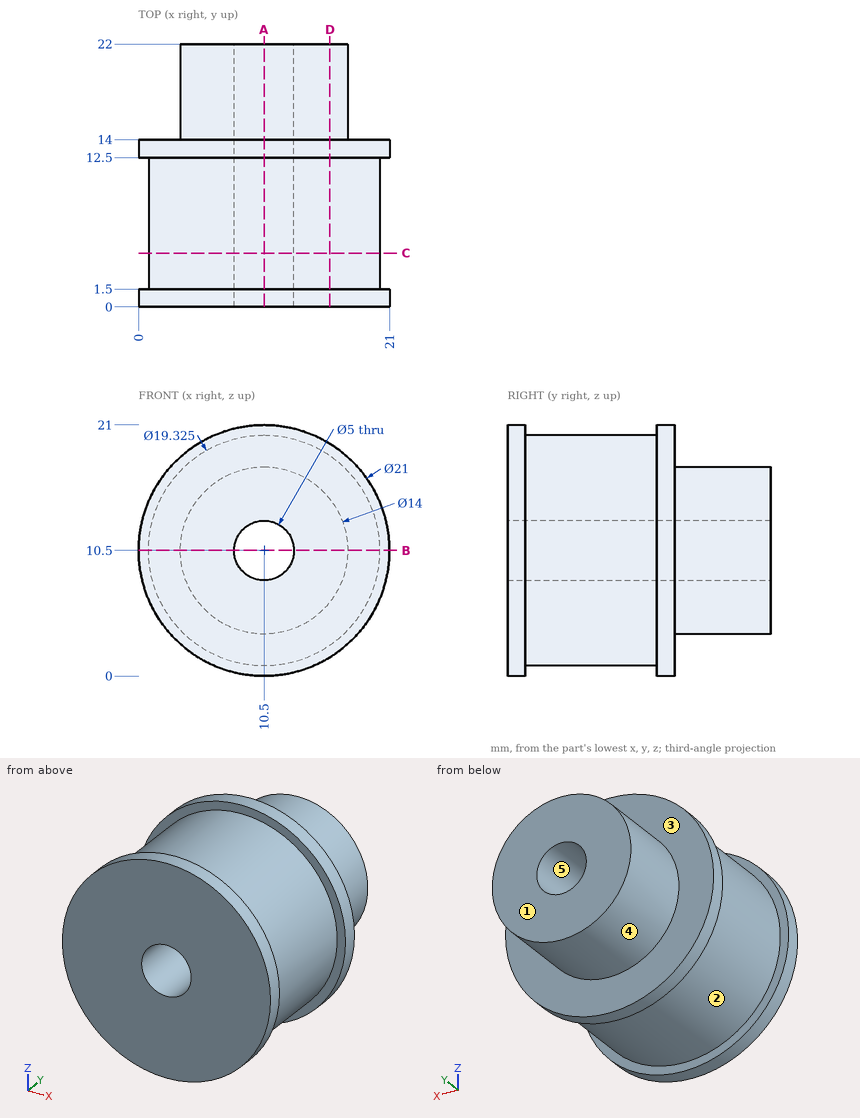
The drawing under review shows one solid part. Ordinate dimensions are in mm from its lowest x, y, z. A direction names the side the tool comes from. Coordinates: 2 decimals unless noted, no trailing zeros. Order: outer loops, then holes, each group sorted by start corner. A loop starts at its lowest first (then second) coordinate and runs counter-clockwise, first axis right, second up. Notation, with made-up numbers: (52, 31.5) -> (56, 31.5) arc R23 cw to (56, 67.5) -> close; hole circle Ø7 at (74.5, 54.25). An arc over 180 degrees is marked (long way). Use CSV: the item, a comma, the result in double quotes. Start each with the question number.
Item 1: We need section A-A, the plane x = 10.5. Give the boundary of the cut face in (y, z).
Item 2: We need section D-D, the plane x = 16. Give the boundary of the cut face in (y, z).
Item 3: We need section C-C, the plane y = 4.5. Give the boundary of the cut face in (x, z) (1 decimal), then the cut area to 3 significant figures.
Item 4: We need section B-B, the plane z = 10.5. Give the boundary of the cut face in (x, y).
Item 5: For the marked faces 1 and 2, list the 3-axis set-ups (+Z, -Z, +X, -X, +Y, -Y) from which the entire face can be reached by the end or side of a thin tool; tool diameter is ignored.
Item 6: Wall thickness on probe 1 along X at (y, z) = (5.25, 10.5); probe 2 along X at (y, z) = (13.25, 10.5); probe 3 along X at (y, z) = (16.5, 14.75): over which ranges is each line inside the solid? List them lowest first.
Item 7: Insertion check: pin 1 (3 mm diameter, centred on y = 10.5, z = 3, fed in from +X); pin 2 (1 mm diameter, centred on x = 11, z = 10, fed in from +Y); pin 3 (8 mm diameter, centred on x = 2.5, y = 17, fed in from -Z); pin 4 (1.5 mm diameter, centred on x = 10.5, y = 8, fed in from -Z). Each pin has a flat end and moves straight along its axis. Give the tip position at first contact, or say it passes through.
Item 8: Draft analysis for pull direction X (two halves, no side actions). For the marked faces 3, 4 and 5, state which applies: pulls with the +X half, pulls with the -X half, needs draft (parallel to the pull), parting line crosses it, or undercut.
Derived:
1,outline,"(0, 0) -> (1.5, 0) -> (1.5, 0.84) -> (12.5, 0.84) -> (12.5, 0) -> (14, 0) -> (14, 3.5) -> (22, 3.5) -> (22, 8) -> (0, 8) -> close; (0, 13) -> (22, 13) -> (22, 17.5) -> (14, 17.5) -> (14, 21) -> (12.5, 21) -> (12.5, 20.16) -> (1.5, 20.16) -> (1.5, 21) -> (0, 21) -> close"
2,outline,"(0, 1.56) -> (1.5, 1.56) -> (1.5, 2.56) -> (12.5, 2.56) -> (12.5, 1.56) -> (14, 1.56) -> (14, 6.17) -> (22, 6.17) -> (22, 14.83) -> (14, 14.83) -> (14, 19.44) -> (12.5, 19.44) -> (12.5, 18.44) -> (1.5, 18.44) -> (1.5, 19.44) -> (0, 19.44) -> close"
3,outline,"circle Ø19.3 at (10.5, 10.5); hole circle Ø5 at (10.5, 10.5)"
3,area,"274 mm^2"
4,outline,"(0, 0) -> (8, 0) -> (8, 22) -> (3.5, 22) -> (3.5, 14) -> (0, 14) -> (0, 12.5) -> (0.84, 12.5) -> (0.84, 1.5) -> (0, 1.5) -> close; (13, 0) -> (21, 0) -> (21, 1.5) -> (20.16, 1.5) -> (20.16, 12.5) -> (21, 12.5) -> (21, 14) -> (17.5, 14) -> (17.5, 22) -> (13, 22) -> close"
5,face 1,"+Z, -Z, +X, -X, +Y"
5,face 2,"none"
6,probe 1,"x = 0.84 to 8, 13 to 20.16"
6,probe 2,"x = 0 to 8, 13 to 21"
6,probe 3,"x = 4.94 to 16.06"
7,pin 1,"stops at x = 18.07"
7,pin 2,"passes through"
7,pin 3,"stops at z = 1.47"
7,pin 4,"stops at z = 0.84"
8,face 3,"needs draft"
8,face 4,"parting line crosses it"
8,face 5,"undercut"
